Job drawing, mm, ordinate dimensions from the low corner. One solid piece. Give positions to 0.01 mm unless a question says otherwise; leave off trailing zeros. Write each loop counter-clockwise with the first axis right and the second up, starting at its lowest first coordinate (ties: lowest second). Pieces come first, ordered by that corner, then holes. Notation, with made-up numbers: M -6,-39 L 29,-39 A17 ccw 29,-19 Z; hole C -20,-17.75 d10. An arc over 180 degrees is marked long. Use CSV: the item, a comma, the result in double quotes. Start each with the question number.
Item 1: Cut at A-A (x = 14). List the corners of the cut face in (y, z).
Item 2: Pin check, flat tips, straight feed: pin 1 (8 mm diameter, centred on x = 21.5, z = 11.5, fed in from +Y); pin 2 (1 mm diameter, centred on y = 2, z = 19.5, fed in from +X); pin 3 (12 mm diameter, centred on x = 14, z = 14, fed in from -Y). Stop position of each tip, or through.
Item 3: Mould opens along X. For the marked faces 1, 2 and 3 say: released by +X, released by -X, zero draft, split by the parting line, or undercut.
Item 4: Cut at C-C (y = 1.3). List the corners of the cut face in (x, z), then the cut area to 3 significant figures.
Item 5: Cut at B-B (z = 14). List the corners of the cut face in (x, y), then the cut area to 3 significant figures.
Item 6: Drill centre lines: line 1 (Z direction, x = 14, y = 1.3); line 2 (Y direction, x = 25, z = 6.25). Where is each one in solid material? Low to high. Write a range as [from, to].
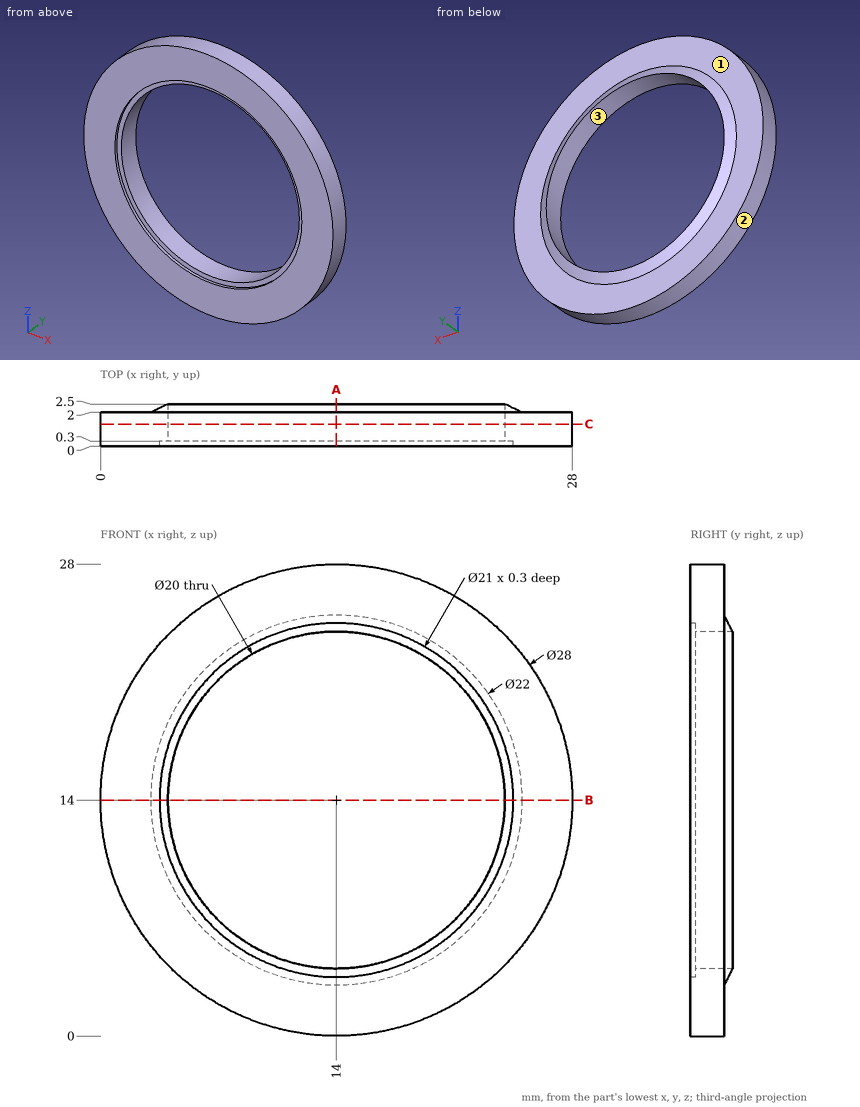
Worked answers:
1,outline,"M 0,0 L 2,0 L 2,3 L 2.5,4 L 0.3,4 L 0.3,3.5 L 0,3.5 Z; M 0,24.5 L 0.3,24.5 L 0.3,24 L 2.5,24 L 2,25 L 2,28 L 0,28 Z"
2,pin 1,"stops at y = 2.5"
2,pin 2,"stops at x = 27.08"
2,pin 3,"passes through"
3,face 1,"zero draft"
3,face 2,"split by the parting line"
3,face 3,"undercut"
4,outline,"C 14,14 d28; hole C 14,14 d20"
4,area,"302 mm^2"
5,outline,"M 0,0 L 3.5,0 L 3.5,0.3 L 4,0.3 L 4,2.5 L 3,2 L 0,2 Z; M 24,0.3 L 24.5,0.3 L 24.5,0 L 28,0 L 28,2 L 25,2 L 24,2.5 Z"
5,area,"16.2 mm^2"
6,line 1,"z = [0, 4], [24, 28]"
6,line 2,"y = [0, 2]"
